Autodesk Inventor part; units mm, degrees
ref_plane "YZ Plane" through (0, 0, 0) normal (1, 0, 0) x (0, 1, 0)
ref_plane "XZ Plane" through (0, 0, 0) normal (0, 1, 0) x (-1, 0, 0)
ref_plane "XY Plane" through (0, 0, 0) normal (0, 0, 1) x (1, 0, 0)
sketch "Sketch4" plane through (0, 0, 0) normal (0, 1, 0) x (-1, 0, 0)
  line L0 (75, -40) -> (-75, -40)
  line L1 (-75, -40) -> (-75, 0)
  line L2 (-75, 0) -> (75, 0)
  line L3 (75, 0) -> (75, -40)
  point P0 (0, 0)
  point P1 (0, 0)
  dimension "d36" = 150
  dimension "d37" = 40
extrude "Plate2" add sketch "Sketch4" along normal blind 3
sketch "Sketch5" plane through (0, 0, 0) normal (0, -1, 0) x (1, 0, 0)
  circle A0 centre (-60, -25) radius 6.5
  circle A1 centre (60, -25) radius 6.5
  line L0 (0, 0) -> (0, -40) construction
  line L1 (75, -40) -> (-75, -40) construction
  dimension "d39" = 120
  dimension "d40" = 15
  dimension "d41" = 13
extrude "Cut1" cut sketch "Sketch5" against normal blind 3
sketch "Sketch6" plane through (-75, 3, -3) normal (0, 0, 1) x (1, 0, 0)
  line L0 (150, 0) -> (0, 0)
  line L1 (0, 0) -> (0, -40)
  line L2 (0, -40) -> (150, -40)
  line L3 (150, -40) -> (150, 0)
edge flange "Flange1" height 40 angle 90 thickness 3 bend radius 5 thickness toward (0, 0, 1) relief round relief width 3 relief depth 1.5 edges at (0, 0, 0) wall of the first edge with corners at (75, 3, -3) (-75, 3, -3) (-75, -37, -3) (75, -37, -3)
bend "Bend1"
corner "Corner1"
fillet "Corner Round6" radius 6 4 edges at (75, -37, -1.5) (-75, 1.5, -40) (75, 1.5, -40) (-75, -37, -1.5)
equation "\"d42\" = Thickness"
equation "\"d38\" = Thickness"
equation "\"d44\" = BendReliefWidth"
equation "\"d45\" = BendReliefDepth"
equation "\"d46\" = MinimumRemnant"
equation "\"d47\" = TransitionRadius"
equation "\"d50\" = BendRadius"
equation "\"d51\" = CornerReliefSize"
equation "\"d52\" = GapSize"
equation "\"d53\" = JacobiRadiusSize"
equation "\"BendReliefWidth\" = Thickness"
equation "\"BendReliefDepth\" = 0.5 * Thickness"
equation "\"CornerReliefSize\" = 4 * Thickness"
equation "\"MinimumRemnant\" = 2 * Thickness"
equation "\"TransitionRadius\" = BendRadius"
equation "\"JacobiRadiusSize\" = BendRadius"
equation "\"GapSize\" = Thickness"
properties part number "NDM-VOS 712 flange" material "Stainless Steel"
Part model, mm, in its own coordinate system. A direction names the side the tool comes from. Give positions to 0.01 mm unless a question says otherwise; leave off trailing zeros. Write each loop counter-clockwise with the first axis right and the second up, starting at its lowest first coordinate (ties: lowest second). Pieces come first, ordered by that corner, then holes.
1) Which spindle directions (+Z, -Z, +X, -X, +Y, -Y) get a long thin tool onto all of the face, cutting with end or side? Do faces 1 (the face through (-1.05, 0.594, -2.281)), 2 (the face through (-1, -21, -3)). Say none if no direction does.
Resolved:
face 1: +Z, +X, -X, +Y
face 2: -Z, +X, -X, -Y
2) Probe L1, parallel to Y at x = 0.5, z = -28; L2, parallel to Z at x = 54.5, y = -15; L3, parallel to Z at x = -60, y = 1. List the from-to ranges inside material, lowest first.
Resolved:
L1: y = 0 to 3
L2: z = -3 to 0
L3: z = -40 to -31.5, -18.5 to -2.71
3) Cut at A-A on z = -25. Write the cut outline in (x, y).
Resolved:
outline: (-75, 0) - (-66.5, 0) - (-66.5, 3) - (-75, 3) - close; (-53.5, 0) - (53.5, 0) - (53.5, 3) - (-53.5, 3) - close; (66.5, 0) - (75, 0) - (75, 3) - (66.5, 3) - close
4) Cut at D-D on y = -29.5. Write the cut outline in (x, z), then the cut area to 3 significant figures.
Resolved:
outline: (-75, -3) - (75, -3) - (75, 0) - (-75, 0) - close
area: 450 mm2
5) Two-plate mould, pull along X, no slides. Class faces 3 (the face through (-73.289, -35.196, -1.479)), 4 (the face through (1, 0, -24)), 5 (the face through (66.2, 1.48, -23.05)): released by +X, released by -X, zero draft, split by the parting line, or undercut.
Resolved:
face 3: released by -X
face 4: zero draft
face 5: undercut
6) Cut at B-B on x = -60. Write the cut outline in (y, z), then the cut area to 3 significant figures.
Resolved:
outline: (-37, -3) - (-5, -3) arc R5 cw to (0, -8) - (0, -18.5) - (3, -18.5) - (3, -8) arc R8 ccw to (-5, 0) - (-37, 0) - close; (0, -40) - (3, -40) - (3, -31.5) - (0, -31.5) - close
area: 184 mm2
7) Cut at C-C on x = 25. Write the cut outline in (y, z), then the cut area to 3 significant figures.
Resolved:
outline: (-37, -3) - (-5, -3) arc R5 cw to (0, -8) - (0, -40) - (3, -40) - (3, -8) arc R8 ccw to (-5, 0) - (-37, 0) - close
area: 223 mm2
8) Pin check, flat tips, straight feed: pin 1 (6 mm diameter, centred on x = -22.5, y = -26, fed in from -Z); pin 2 (1 mm diameter, centred on x = 5, y = -1.5, fed in from +Z); pin 3 (10 mm diameter, centred on x = -42.5, y = -31, fed in from +Z); pin 4 (9.5 mm diameter, centred on x = -28, z = -19, fed in from -Y). Stop position of each tip, or through.
Resolved:
pin 1: stops at z = -3
pin 2: stops at z = -0.58
pin 3: stops at z = 0
pin 4: stops at y = 0
